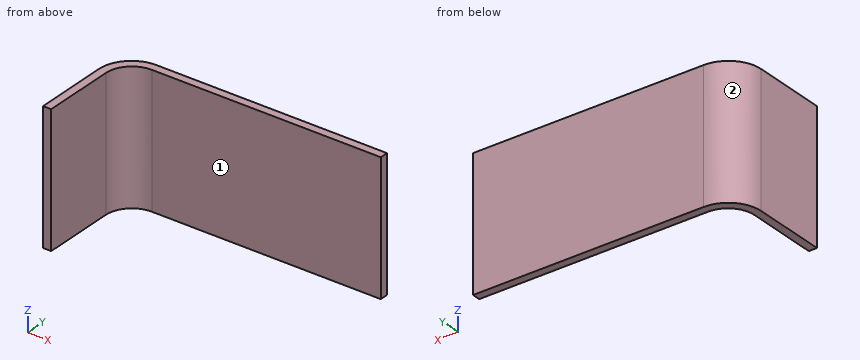
```python
from build123d import *

# Parameters (mm, degrees)
BOSS_EXTRUDE1_DEPTH = 101.6


with BuildPart() as part:
    # Sketch1 → Boss-Extrude1 (new body)
    with BuildSketch(Plane.XY):
        with BuildLine():
            Line((25.4, 0), (204.47, 0))
            Line((204.47, 0), (204.47, -6.35))
            Line((204.47, -6.35), (26.67, -6.35))
            ThreePointArc((26.67, -6.35), (12.301590206, -12.301590206), (6.35, -26.67))
            Line((6.35, -26.67), (6.35, -82.55))
            Line((6.35, -82.55), (0, -82.55))
            Line((0, -82.55), (0, -25.4))
            ThreePointArc((0, -25.4), (7.439487758, -7.439487758), (25.4, 0))
        make_face()
    extrude(amount=BOSS_EXTRUDE1_DEPTH)


solid = part.part
```
Input: part model. Units: mm. Frame: model coordinates. Face numbers are marked on the shaded views. A direction names the side the tool comes from. Give positions to 0.01 mm unless a question says otherwise; leave off trailing zeros. Order: outer loops, then holes, each group sorted by start corner. A loop starts at its lowest first (then second) coordinate and runs counter-clockwise, first axis right, second up.
1. Pin query (flat end, axial travel): pin 1 Ø1.5 at (y, z) = (-15, 68) entering from -X; pin 2 Ø4 at (x, z) = (141, 54.5) entering from -Y. Return the tip coordinate at first contact, or that it passes through.
Computed:
pin 1: stops at x = 1.9
pin 2: stops at y = -6.35
2. Cut plane A-A (z = 29). Return loops of the section in (x, y), and give its area (3 significant figures).
Computed:
outline: (0, -82.55) - (6.35, -82.55) - (6.35, -26.67) arc R20.32 cw to (26.67, -6.35) - (204.47, -6.35) - (204.47, 0) - (25.4, 0) arc R25.4 ccw to (0, -25.4) - close
area: 1,730 mm2
3. Cut plane B-B (x = 132.5). Return loops of the section in (y, z), and give its area (3 significant figures).
Computed:
outline: (-6.35, 0) - (0, 0) - (0, 101.6) - (-6.35, 101.6) - close
area: 645 mm2
4. Cut plane C-C (y = -72.5). Return loops of the section in (x, z).
Computed:
outline: (0, 0) - (6.35, 0) - (6.35, 101.6) - (0, 101.6) - close
5. Set-up query: the marked faces 1 and 2. Return all of +Z, -Z, +X, -X, +Y, -Y with unobstructed straight access to the full face (end or side cutting, diameter ignored); none if empty.
Computed:
face 1: +Z, -Z, +X, -Y
face 2: +Z, -Z, -X, +Y
6. Line query: probe 1 along X at (y, z) = (-55, 49); probe 2 along Y at (x, z) = (62.5, 11). Output: solid intervals per line, ascending.
Computed:
probe 1: x = 0 to 6.35
probe 2: y = -6.35 to 0
